Geometry: final body of the model. Coordinates: model frame, mm. A direction names the side the tool comes from. Give positions to 0.01 mm unless a question says otherwise; leave off trailing zeros. Order: outer loops, then holes, each group sorted by start corner. A loop starts at its lowest first (then second) coordinate and runs counter-clockwise, first axis right, second up. Notation, with made-up numbers: (82.25, -10) - (91.25, -10) arc R35 cw to (91.25, 22) - close; hole circle Ø6 at (65, 82.25). An arc over 180 degrees is marked (long way). Use one line per item in the form item = value.
from build123d import *

# Parameters (mm, degrees)
F1_DEPTH = 63.5
F2_DEPTH = 127
F3_DEPTH = 63.5
F4_W     = 63.5
F4_H     = 31.75
F5_DEPTH = 101.6
F6_DEPTH = 190.501


with BuildPart() as f1:
    # F0 (on Front) → F1 (new body)
    with BuildSketch(Plane.XZ):
        Polygon((-158.75, -31.75), (-158.75, -95.25), (158.75, -95.25), (158.75, 95.25), (95.25, 95.25), (95.25, 44.45), (31.75, -6.35), (31.75, 69.85), (-31.75, 69.85), (-31.75, -6.35), (-95.25, -6.35), (-95.25, -31.75), align=None)
        Polygon((95.25, 44.45), (95.25, 95.25), (-95.25, 95.25), (-95.25, -6.35), (-31.75, -6.35), (-31.75, 69.85), (31.75, 69.85), (31.75, -6.35), align=None)
        Polygon((-158.75, 95.25), (-158.75, -31.75), (-95.25, -31.75), (-95.25, -6.35), (-95.25, 95.25), align=None)
    extrude(amount=-F1_DEPTH)

    # F0 (on Front) → F2 (join)
    with BuildSketch(Plane.XZ):
        Polygon((-158.75, 95.25), (-158.75, -31.75), (-95.25, -31.75), (-95.25, -6.35), (-95.25, 95.25), align=None)
    extrude(amount=F2_DEPTH)

    # F0 (on Front) → F3 (join)
    with BuildSketch(Plane.XZ):
        Polygon((95.25, 44.45), (95.25, 95.25), (-95.25, 95.25), (-95.25, -6.35), (-31.75, -6.35), (-31.75, 69.85), (31.75, 69.85), (31.75, -6.35), align=None)
    extrude(amount=F3_DEPTH)

    # F4 (on face) → F5 (cut)
    with BuildSketch(Plane(origin=(0, 0, -95.25), x_dir=(1, 0, 0), z_dir=(0, 0, -1))):
        with Locations((127, -47.625)):
            Rectangle(F4_W, F4_H)
    extrude(amount=-F5_DEPTH, mode=Mode.SUBTRACT)

    # F4 (on face) → F6 (cut, through all)
    with BuildSketch(Plane(origin=(0, 0, -95.25), x_dir=(1, 0, 0), z_dir=(0, 0, -1))):
        with Locations((-31.75, -47.625)):
            Rectangle(F4_W, F4_H)
    extrude(amount=-F6_DEPTH, mode=Mode.SUBTRACT)


solid = f1.part
(1) Pull-direction query (X, two-part tool) for faces 4 (the face through (0, 48, -1)), 5 (the face through (127, 31.75, -45)), 6 (the face through (95.25, -31, 69)); classes: released by +X, released by -X, zero draft, split by the parting line, or undercut.
Computed values:
face_4 = undercut
face_5 = zero draft
face_6 = released by +X
(2) Ray query, line 1 along X through (y, z) = (-52.5, 65.5); line 2 along X through (y, z) = (39.5, 31.5); line 3 along Z through (x, y) = (-23, -27). Return the intervals inside material, ascending.
Computed values:
line_1 = -158.75 to -31.75, 31.75 to 95.25
line_2 = -158.75 to -63.5, 0 to 158.75
line_3 = 69.85 to 95.25
(3) Cut plane A-A on y = 52.5. Output: boundary loops of the cut face in (x, z).
Computed values:
outline = (-158.75, -95.25) - (-63.5, -95.25) - (-63.5, 95.25) - (-158.75, 95.25) - close; (0, -95.25) - (95.25, -95.25) - (95.25, 6.35) - (158.75, 6.35) - (158.75, 95.25) - (0, 95.25) - close
(4) Cut plane B-B on z = -56.5. Output: boundary loops of the cut face in (x, y).
Computed values:
outline = (-158.75, 0) - (158.75, 0) - (158.75, 31.75) - (95.25, 31.75) - (95.25, 63.5) - (0, 63.5) - (0, 31.75) - (-63.5, 31.75) - (-63.5, 63.5) - (-158.75, 63.5) - close
(5) Cut plane C-C on x = 19.5. Output: boundary loops of the cut face in (y, z), plus the area to 3 significant figures.
Computed values:
outline = (-63.5, 69.85) - (0, 69.85) - (0, -95.25) - (63.5, -95.25) - (63.5, 95.25) - (-63.5, 95.25) - close
area = 13,700 mm²
(6) Reachability of faces 1 (the face through (63.056, -31.306, 18.694)), 2 (the face through (0, -31, 69.85)), 3 (the face through (-32, 31.75, -1)) from +Z, -Z, +X, -X, +Y, -Y: full face, straight path, thin tool, end or side. Return the list, or none.
Computed values:
face_1 = -Z, +X, -Y
face_2 = -Z, -Y
face_3 = +Z, -Z, +Y
(7) Cut plane D-D on y = -25. Output: boundary loops of the cut face in (x, z).
Computed values:
outline = (-158.75, -31.75) - (-95.25, -31.75) - (-95.25, -6.35) - (-31.75, -6.35) - (-31.75, 69.85) - (31.75, 69.85) - (31.75, -6.35) - (95.25, 44.45) - (95.25, 95.25) - (-158.75, 95.25) - close
(8) Contact query for flat-ended pins moving along their axis: pin 1 Ø19 at (y, z) = (-18.5, 46) entering from +X; pin 2 Ø1.5 at (y, z) = (-79.5, 45.5) entering from +X; pin 3 Ø5 at (x, y) = (46, -45) entering from -Z. Output: stop coordinate, or through.
Computed values:
pin_1 = 95.25
pin_2 = -95.25
pin_3 = 3.05
